from build123d import *

# Parameters (mm, degrees)
SKETCH1_W           = 44.45
SKETCH1_H           = 38.1
BOSS_EXTRUDE1_DEPTH = 12.7
SKETCH4_W           = 44.45
SKETCH4_H           = 11.16076
CUT_EXTRUDE1_DEPTH  = 108.033044593
SKETCH5_R           = 6.35
BOSS_EXTRUDE2_DEPTH = 12.7


with BuildPart() as part:
    # Sketch1 → Boss-Extrude1 (new body)
    with BuildSketch(Plane(origin=(0, 0, 0), x_dir=(1, 0, 0), z_dir=(0, 1, 0))):
        with Locations((-76.987764476, 18.013859456)):
            Rectangle(SKETCH1_W, SKETCH1_H)
    extrude(amount=BOSS_EXTRUDE1_DEPTH)

    # Sketch4 → Cut-Extrude1 (cut, through all)
    with BuildSketch(Plane(origin=(0, 0, -37.063859456), x_dir=(-1, 0, 0), z_dir=(0, 0, -1))):
        with Locations((76.987764476, 7.11962)):
            Rectangle(SKETCH4_W, SKETCH4_H)
    extrude(amount=-CUT_EXTRUDE1_DEPTH, mode=Mode.SUBTRACT)

    # Sketch5 → Boss-Extrude2 (add)
    with BuildSketch(Plane(origin=(0, 1.53924, 0), x_dir=(1, 0, 0), z_dir=(0, 1, 0))):
        with Locations(Location((-89.052764476, 18.013859456, 0), (0, 0, 270))):
            Circle(SKETCH5_R)
    extrude(amount=BOSS_EXTRUDE2_DEPTH)


solid = part.part
Could you check a few things on this model? Use its own coordinates, in mm. A direction names the side the tool comes from. Round coordinates to 2 decimals unless told otherwise and drop trailing zeros. Write each loop counter-clockwise with the first axis right and the second up, starting at its lowest first coordinate (ties: lowest second). Pieces come first, ordered by that corner, then holes. Notation, with made-up numbers: (10.25, 55) - (52.25, 55) arc R12 cw to (52.25, 69) - close; hole circle Ø9 at (-14.75, 43.5). An arc over 180 degrees is marked (long way). Put each result on its own line as item: value. Start each with the question number.
(1) I want a section at C-C, the plane y = 3.75. Please give me the cut outline in (x, z), plus the area to 3 significant figures.
(2) I want a section at B-B, the plane z = -22.5. Please give me the cut outline in (x, y).
(3) I need wall thicknesses on probe 1 along Y at (x, z) = (-80.5, -14); probe 2 along X at (y, z) = (7, -18); probe 3 along X at (y, z) = (5, -17). Which ranges of each line are inside material? Lowest first, please.
(4) For faces 1 (the flat face through (-77, 1, -37.064)), 2 (the cylindrical face through (-82.757, 7.8, -18.841)), which set-ups out of +Z, -Z, +X, -X, +Y, -Y let a thin tool reach every point of the face, with its end or its side?
(5) I want a section at A-A, the plane x = -85.5. Please give me the cut outline in (y, z).
(6) I want a section at D-D, the plane z = -34. Please give me the cut outline in (x, y), plus the area to 3 significant figures.
Here are the results:
1. outline: circle Ø12.7 at (-89.05, -18.01)
1. area: 127 mm^2
2. outline: (-99.21, 0) - (-54.76, 0) - (-54.76, 1.54) - (-84.56, 1.54) - (-84.56, 14.24) - (-93.55, 14.24) - (-93.55, 1.54) - (-99.21, 1.54) - close
3. probe 1: y = 0 to 1.54
3. probe 2: x = -95.4 to -82.7
3. probe 3: x = -95.32 to -82.78
4. face 1: -Z, +X, -X, +Y, -Y
4. face 2: +Y
5. outline: (0, -37.06) - (1.54, -37.06) - (1.54, -23.28) - (14.24, -23.28) - (14.24, -12.75) - (1.54, -12.75) - (1.54, 1.04) - (0, 1.04) - close
6. outline: (-99.21, 0) - (-54.76, 0) - (-54.76, 1.54) - (-99.21, 1.54) - close
6. area: 68.4 mm^2
